Geometry check sheet. Reference: the model listing, model coordinates, mm. A direction names the side the tool comes from. Round coordinates to 2 decimals unless told otherwise and drop trailing zeros. Write each loop counter-clockwise with the first axis right and the second up, starting at its lowest first coordinate (ties: lowest second). Pieces come first, ordered by that corner, then holes. Notation, with made-up numbers: (81.5, 46) -> (97.5, 46) arc R27 ccw to (97.5, 70) -> close; hole circle Ø6 at (63, -20). An arc over 180 degrees is marked (long way). One line per question, with ' | ' between items.
```python
from build123d import *

# Parameters (mm, degrees)
SKETCH1_W           = 12.7
SKETCH1_H           = 9.525
BOSS_EXTRUDE1_DEPTH = 12.7
SKETCH2_R           = 1.1303
CUT_EXTRUDE1_DEPTH  = 6.35
SKETCH3_W           = 21.59
SKETCH3_H           = 9.525
BOSS_EXTRUDE2_DEPTH = 6.35
SKETCH4_R           = 1.1303
CUT_EXTRUDE2_DEPTH  = 6.35


with BuildPart() as part:
    # Sketch1 → Boss-Extrude1 (new body)
    with BuildSketch(Plane(origin=(0, 0, 0), x_dir=(1, 0, 0), z_dir=(0, 1, 0))):
        Rectangle(SKETCH1_W, SKETCH1_H)
    extrude(amount=BOSS_EXTRUDE1_DEPTH)

    # Sketch2 → Cut-Extrude1 (cut)
    with BuildSketch(Plane(origin=(0, 12.7, 0), x_dir=(1, 0, 0), z_dir=(0, 1, 0))):
        with Locations((-3.175, 0)):
            Circle(SKETCH2_R)
        with Locations((3.175, 0)):
            Circle(SKETCH2_R)
    extrude(amount=-CUT_EXTRUDE1_DEPTH, mode=Mode.SUBTRACT)

    # Sketch3 → Boss-Extrude2 (add)
    with BuildSketch(Plane.XZ):
        Rectangle(SKETCH3_W, SKETCH3_H)
    extrude(amount=BOSS_EXTRUDE2_DEPTH)

    # Sketch4 → Cut-Extrude2 (cut)
    with BuildSketch(Plane.XZ.offset(6.35)):
        with Locations((-4.7625, 0)):
            Circle(SKETCH4_R)
        with Locations((4.7625, 0)):
            Circle(SKETCH4_R)
    extrude(amount=-CUT_EXTRUDE2_DEPTH, mode=Mode.SUBTRACT)


solid = part.part
```
(1) Material ranges on line 1 (X direction, y = 8, z = 0); line 2 (Y direction, x = 10.25, z = 0.25); line 3 (X direction, y = 10.25, z = 2.25), recorded low to high.
Resolved:
line 1: x = -6.35 to -4.31, -2.04 to 2.04, 4.31 to 6.35 | line 2: y = -6.35 to 0 | line 3: x = -6.35 to 6.35
(2) Sectioned sample at C-C on y = 0.5. Record the cut outline in (x, z), then the cut area to 3 significant figures.
Resolved:
outline: (-6.35, -4.76) -> (6.35, -4.76) -> (6.35, 4.76) -> (-6.35, 4.76) -> close | area: 121 mm2
(3) Access from +Z, -Z, +X, -X, +Y, -Y to the whole of each face (thin tool, end or side, straight path). Record for faces 1 (the flat face through (-9, 0, 0)), 2 (the cylindrical face through (2.046, 9.569, -0.05)), 3 (the flat face through (-5, 0, 0)).
Resolved:
face 1: +Z, -Z, -X, +Y | face 2: +Y | face 3: -Y
(4) Sectioned sample at A-A on z = -3.5. Record the cut outline in (x, y) (3 decimals), then the cut area to 3 significant figures.
Resolved:
outline: (-10.795, -6.35) -> (10.795, -6.35) -> (10.795, 0) -> (6.35, 0) -> (6.35, 12.7) -> (-6.35, 12.7) -> (-6.35, 0) -> (-10.795, 0) -> close | area: 298 mm2
(5) Sectioned sample at D-D on z = 0.5. Record the cut outline in (x, y) (3 decimals), then the cut area to 3 significant figures.
Resolved:
outline: (-10.795, -6.35) -> (-5.776, -6.35) -> (-5.776, 0) -> (-3.749, 0) -> (-3.749, -6.35) -> (3.749, -6.35) -> (3.749, 0) -> (5.776, 0) -> (5.776, -6.35) -> (10.795, -6.35) -> (10.795, 0) -> (6.35, 0) -> (6.35, 12.7) -> (4.189, 12.7) -> (4.189, 6.35) -> (2.161, 6.35) -> (2.161, 12.7) -> (-2.161, 12.7) -> (-2.161, 6.35) -> (-4.189, 6.35) -> (-4.189, 12.7) -> (-6.35, 12.7) -> (-6.35, 0) -> (-10.795, 0) -> close | area: 247 mm2
(6) Draft check along X on faces 4 (the flat face through (10.795, -3, 0)), 5 (the flat face through (-6.35, 6, 0)), 6 (the flat face through (-3, 6.35, 0)), 7 (the cylindrical face through (5.84, -3.22, 0.34)). Enter one of: +X half, -X half, draft (parallel to the pull), parting line (faces both ways), or undercut.
Resolved:
face 4: +X half | face 5: -X half | face 6: undercut | face 7: undercut
(7) Go/stop test with flat-tipped pins: pin 1 (1.4 mm diameter, centred on x = -3.175, z = 0, fed in from +Y); pin 2 (1.5 mm diameter, centred on y = 4.5, z = -1, fed in from -X); pin 3 (1.3 mm diameter, centred on x = -9, z = -2, fed in from +Y). Record where each tip stops, or that it passes through.
Resolved:
pin 1: stops at y = 6.35 | pin 2: stops at x = -6.35 | pin 3: stops at y = 0
(8) Sectioned sample at B-B on y = 6.75. Count the separate pieces of the cut face and the enclosed holes in it, then the cut area to 3 significant figures.
Resolved:
separate pieces: 1 | enclosed holes: 2 | area: 113 mm2
